Autodesk Inventor part; units mm, degrees
ref_plane "YZ Plane" through (0, 0, 0) normal (1, 0, 0) x (0, 1, 0)
ref_plane "XZ Plane" through (0, 0, 0) normal (0, 1, 0) x (-1, 0, 0)
ref_plane "XY Plane" through (0, 0, 0) normal (0, 0, 1) x (1, 0, 0)
sketch "スケッチ1" plane through (0, 0, 0) normal (0, 0, 1) x (1, 0, 0)
  line L0 (-37.5496, 23.6801) -> (-7.5496, 23.6801)
  line L1 (3.4504, 19.2991) -> (3.4504, -3.9388)
  line L2 (-7.5496, -8.3199) -> (-37.5496, -8.3199)
  line L3 (-39.5496, -6.3199) -> (-39.5496, 21.6801)
  circle A0 centre (-36.8093, -5.8199) radius 1.05
  circle A1 centre (-36.8093, 21.1801) radius 1.05
  arc A2 (-37.5496, 23.6801) -> (-39.5496, 21.6801) centre (-37.5496, 21.6801) ccw
  arc A3 (-39.5496, -6.3199) -> (-37.5496, -8.3199) centre (-37.5496, -6.3199) ccw
  circle A4 centre (-9.8093, -5.8199) radius 1.05
  circle A5 centre (-9.8093, 21.1801) radius 1.05
  line L4 (-39.5496, 7.6801) -> (3.4504, 7.6801) construction
  line L5 (-17.0496, 23.6801) -> (-17.0496, -8.3199) construction
  arc A6 (-7.5496, -8.3199) -> (3.4504, -3.9388) centre (-7.5496, 7.6801) ccw
  arc A7 (3.4504, 19.2991) -> (-7.5496, 23.6801) centre (-7.5496, 7.6801) ccw
  point P0 (-39.5496, -8.3199)
  point P1 (-17.0496, 7.6801)
  dimension "d23" = 2.1
  dimension "d24" = 2.1
  dimension "d25" = 27
  dimension "d26" = 2.5
  dimension "d27" = 2.5
  dimension "d28" = 2
  dimension "d31" = 2.1
  dimension "d32" = 2.1
  dimension "d33" = 27
  dimension "d34" = 27
extrude "押し出し1" add sketch "スケッチ1" along normal blind 32.5
sketch "スケッチ2" plane through (0, 0, 32.5) normal (0, 0, 1) x (1, 0, 0)
  circle A0 centre (-9.8093, 21.1801) radius 1.05
  circle A1 centre (-9.8093, -5.8199) radius 1.05
  circle A2 centre (-36.8093, 21.1801) radius 1.05
  circle A3 centre (-36.8093, -5.8199) radius 1.05
  line L0 (3.4504, -3.9388) -> (3.4504, 19.2991)
  arc A4 (3.4504, 19.2991) -> (-7.5496, 23.6801) centre (-7.5496, 7.6801) ccw
  line L1 (-7.5496, 23.6801) -> (-37.5496, 23.6801)
  arc A5 (-37.5496, 23.6801) -> (-39.5496, 21.6801) centre (-37.5496, 21.6801) ccw
  line L2 (-39.5496, 21.6801) -> (-39.5496, -6.3199)
  arc A6 (-39.5496, -6.3199) -> (-37.5496, -8.3199) centre (-37.5496, -6.3199) ccw
  line L3 (-37.5496, -8.3199) -> (-7.5496, -8.3199)
  arc A7 (-7.5496, -8.3199) -> (3.4504, -3.9388) centre (-7.5496, 7.6801) ccw
  line L4 (-39.5496, 21.6801) -> (-39.5496, -6.3199) construction
  line L5 (-39.5496, 7.6801) -> (3.4504, 7.6801) construction
  line L6 (-7.5496, -8.3199) -> (-37.5496, -8.3199) construction
  line L7 (-18.0496, -8.3199) -> (-18.0496, 23.6801) construction
  line L8 (-7.5496, 23.6801) -> (-37.5496, 23.6801) construction
  circle A8 centre (-8.55, 7.6801) radius 2.7
  circle A9 centre (-8.55, 7.6801) radius 1.3
  point P0 (0, 0)
  dimension "d49" = 5.4
  dimension "d50" = 2.6
  dimension "d51" = 9.4996
extrude "押し出し3" add sketch "スケッチ2" along normal blind 3.5 contours A8
sketch "スケッチ3" plane through (0, 0, 0) normal (0, 0, -1) x (-1, 0, 0)
  circle A0 centre (9.8093, 21.1801) radius 1.05
  circle A1 centre (9.8093, -5.8199) radius 1.05
  circle A2 centre (36.8093, 21.1801) radius 1.05
  circle A3 centre (36.8093, -5.8199) radius 1.05
  line L0 (-3.4504, 19.2991) -> (-3.4504, -3.9388)
  arc A4 (-3.4504, -3.9388) -> (7.5496, -8.3199) centre (7.5496, 7.6801) ccw
  line L1 (7.5496, -8.3199) -> (37.5496, -8.3199)
  arc A5 (37.5496, -8.3199) -> (39.5496, -6.3199) centre (37.5496, -6.3199) ccw
  line L2 (39.5496, -6.3199) -> (39.5496, 21.6801)
  arc A6 (39.5496, 21.6801) -> (37.5496, 23.6801) centre (37.5496, 21.6801) ccw
  line L3 (37.5496, 23.6801) -> (7.5496, 23.6801)
  arc A7 (7.5496, 23.6801) -> (-3.4504, 19.2991) centre (7.5496, 7.6801) ccw
  line L4 (39.5496, -6.3199) -> (39.5496, 21.6801) construction
  line L5 (39.5496, 7.6801) -> (-3.4504, 7.6801) construction
  line L6 (-3.4504, 19.2991) -> (-3.4504, -3.9388) construction
  line L7 (7.5496, -8.3199) -> (37.5496, -8.3199) construction
  line L8 (18.0496, -8.3199) -> (18.0496, 23.6801) construction
  line L9 (37.5496, 23.6801) -> (7.5496, 23.6801) construction
  circle A8 centre (8.55, 7.6801) radius 1.3
  circle A9 centre (31.5496, -5.8199) radius 1.05
  circle A10 centre (18.5496, 21.1801) radius 1.05
  circle A11 centre (1.0496, 18.3126) radius 1.05
  circle A12 centre (1.0496, -3.6874) radius 1.05
  point P0 (0, 0)
  dimension "d54" = 2.6
  dimension "d55" = 2.1
  dimension "d56" = 13.5
  dimension "d57" = 2.1
  dimension "d58" = 0.5
  dimension "d59" = 2.1
  dimension "d60" = 17
  dimension "d61" = 2.1
  dimension "d62" = 22
  dimension "d63" = 17
extrude "押し出し4" cut sketch "スケッチ3" against normal blind 10 contours A8 | A9 | A10 | A11 | A12
sketch "スケッチ4" plane through (-37.5496, -8.3199, 0) normal (0, -1, 0) x (1, 0, 0)
  line L0 (30, 0) -> (0, 0)
  line L1 (30, 0) -> (30, 32.5)
  line L2 (0, 32.5) -> (30, 32.5)
  line L3 (0, 0) -> (0, 32.5)
  line L4 (0, 0) -> (-2, 0)
  line L5 (0, 0) -> (0, 32.5)
  line L6 (-2, 32.5) -> (0, 32.5)
  line L7 (-2, 0) -> (-2, 32.5)
  line L8 (41, 0) -> (30, 0)
  line L9 (41, 0) -> (41, 32.5)
  line L10 (30, 32.5) -> (41, 32.5)
  line L11 (30, 0) -> (30, 32.5)
  line L12 (0, 32.5) -> (30, 32.5) construction
  line L13 (19.5, 32.5) -> (19.5, 0) construction
  line L14 (17.5, 10.5) -> (25.5, 10.5)
  line L15 (25.5, 10.5) -> (25.5, 5)
  line L16 (25.5, 5) -> (17.5, 5)
  line L17 (17.5, 5) -> (17.5, 10.5)
  point P0 (37.5496, 0)
  dimension "d66" = 21.5
  dimension "d67" = 8
  dimension "d68" = 5.5
  dimension "d69" = 5
  dimension "d70" = 2
extrude "押し出し5" add sketch "スケッチ4" along normal blind 3 contours L14 L15 L16 L17
properties part number "KRS-4034HV" material "アセタール樹脂、黒"
Verification items for the finished model (mm, model axes). A direction names the side the tool comes from. Give positions to 0.01 mm unless a question says otherwise; leave off trailing zeros. Order: outer loops, then holes, each group sorted by start corner. A loop starts at its lowest first (then second) coordinate and runs counter-clockwise, first axis right, second up. Notation, with made-up numbers: M 27.25,42 L 80.25,42 A24 cw 80.25,65 Z; hole C 59,89 d11. An arc over 180 degrees is marked long. Return JSON: item names as keys, results as strings. Group by question number.
1) Scan lines: line 1 (X direction, y = 21, z = 29.5); line 2 (X direction, y = -5, z = 29); line 3 (Z direction, x = -19.5, y = 10.5). Record each from-to range of solid material in increasing order.
2) Access from +Z, -Z, +X, -X, +Y, -Y to the whole of each face (thin tool, end or side, straight path). Record for faces 4 (the face through (-6.056, 8.714, 34.226)), 5 (the face through (-16, -10, 5)), 6 (the face through (-1, 18, 10)).
3) Mould release check, pull along Y, two halves, no side actions. Record for faces 1 (the face through (-19.11, 22.07, 4.93)), 2 (the face through (-38.98, 23.08, 16.02)), 3 (the face through (-7, 8, 36)): pulls with the +Y half, pulls with the -Y half, needs draft (parallel to the pull), parting line crosses it, or undercut.
4) Section check A-A on z = 8. Give the number of separate pieces and of enclosed holes in the cut face, and give its area (3 significant figures).
5) Section check B-B on z = 29.5. Record the cut outline in (x, y).
6) Go/stop test with flat-tipped pins: pin 1 Ø2 at (x, z) = (-6.5, 17) entering from -Y; pin 2 Ø0.9 at (y, z) = (-10, 7.5) entering from +X; pin 3 Ø0.9 at (x, y) = (-17, -10.5) entering from +Z. Record where each tip stops, or that it passes through.
7) Section check C-C on x = -27. Record the cut outline in (y, z).
Answer block:
{
 "1": {"line 1": "x = -39.55 to -37.84, -35.77 to -10.84, -8.77 to 1.32", "line 2": "x = -39.55 to -37.47, -36.15 to -10.47, -9.15 to 2.21", "line 3": "z = 0 to 32.5"},
 "2": {"face 4": "+Z", "face 5": "-Z, +X, -X, -Y", "face 6": "-Z"},
 "3": {"face 1": "undercut", "face 2": "pulls with the +Y half", "face 3": "needs draft"},
 "4": {"separate pieces": "1", "enclosed holes": "9", "area": "1,340 mm^2"},
 "5": {"outline": "M -39.55,-6.32 A2 ccw -37.55,-8.32 L -7.55,-8.32 A16 ccw 3.45,-3.94 L 3.45,19.3 A16 ccw -7.55,23.68 L -37.55,23.68 A2 ccw -39.55,21.68 Z; hole C -36.81,-5.82 d2.1; hole C -36.81,21.18 d2.1; hole C -9.81,-5.82 d2.1; hole C -9.81,21.18 d2.1"},
 "6": {"pin 1": "stops at y = -8.32", "pin 2": "stops at x = -12.05", "pin 3": "stops at z = 10.5"},
 "7": {"outline": "M -8.32,0 L 23.68,0 L 23.68,32.5 L -8.32,32.5 Z"}
}
